```python
from build123d import *

# Parameters (mm, degrees)
SALIENTE_EXTRUIR1_DEPTH = 6
SALIENTE_EXTRUIR4_DEPTH = 141
SALIENTE_EXTRUIR5_DEPTH = 6
REDONDEO10_R            = 2
REDONDEO11_R            = 2
CROQUIS8_R              = 5.2625
CORTAR_EXTRUIR5_DEPTH   = 161
CORTAR_EXTRUIR4_DEPTH   = 45.2325
CROQUIS10_W             = 37.37553938
CROQUIS10_H             = 2.5
SALIENTE_EXTRUIR6_DEPTH = 142
CROQUIS15_W             = 31.064336603
CROQUIS15_H             = 2.5
SALIENTE_EXTRUIR8_DEPTH = 148
CROQUIS16_R             = 1.5
CORTAR_EXTRUIR6_DEPTH   = 156
CORTAR_EXTRUIR7_DEPTH   = 64
CROQUIS19_W             = 16.749018002
CROQUIS19_H             = 43
CORTAR_EXTRUIR9_DEPTH   = 157
REDONDEO12_R            = 10


with BuildPart() as part:
    # Croquis1 → Saliente-Extruir1 (new body)
    with BuildSketch(Plane.XY):
        with BuildLine():
            Line((47.278265355, -15.875), (82.039783357, -15.875))
            Line((82.039783357, -15.875), (82.039783357, 30.125))
            Line((82.039783357, 30.125), (40.807283357, 30.125))
            ThreePointArc((40.807283357, 30.125), (38.163219926, 28.542366774), (38.308878254, 25.464285714))
            ThreePointArc((38.308878254, 25.464285714), (45.409629872, 7.346122436), (44.38367768, -12.086734694))
            ThreePointArc((44.38367768, -12.086734694), (44.89448727, -14.696428571), (47.278265355, -15.875))
        make_face()
    extrude(amount=SALIENTE_EXTRUIR1_DEPTH)

    # Croquis6 → Saliente-Extruir4 (add)
    with BuildSketch(Plane(origin=(0, 0, 0), x_dir=(-1, 0, 0), z_dir=(0, 0, -1))):
        with BuildLine():
            Line((-45.807283357, 27.125), (-40.807283357, 27.125))
            ThreePointArc((-40.807283357, 27.125), (-48.371127473, 7.825217377), (-47.278265355, -12.875))
            Line((-47.278265355, -12.875), (-52.278265355, -12.875))
            Line((-52.278265355, -12.875), (-52.278265355, -15.875))
            Line((-52.278265355, -15.875), (-47.278265355, -15.875))
            ThreePointArc((-47.278265355, -15.875), (-44.89448727, -14.696428571), (-44.38367768, -12.086734694))
            ThreePointArc((-44.38367768, -12.086734694), (-45.409629872, 7.346122436), (-38.308878254, 25.464285714))
            ThreePointArc((-38.308878254, 25.464285714), (-38.163219926, 28.542366774), (-40.807283357, 30.125))
            Line((-40.807283357, 30.125), (-45.807283357, 30.125))
            Line((-45.807283357, 30.125), (-45.807283357, 27.125))
        make_face()
    extrude(amount=SALIENTE_EXTRUIR4_DEPTH)

    # Croquis7 → Saliente-Extruir5 (add)
    with BuildSketch(Plane(origin=(0, 0, -141), x_dir=(-1, 0, 0), z_dir=(0, 0, -1))):
        with BuildLine():
            Line((-82.039783357, 30.125), (-40.807283357, 30.125))
            ThreePointArc((-40.807283357, 30.125), (-38.163219926, 28.542366774), (-38.308878254, 25.464285714))
            ThreePointArc((-38.308878254, 25.464285714), (-45.409629872, 7.346122436), (-44.38367768, -12.086734694))
            ThreePointArc((-44.38367768, -12.086734694), (-44.89448727, -14.696428571), (-47.278265355, -15.875))
            Line((-47.278265355, -15.875), (-82.039783357, -15.875))
            Line((-82.039783357, -15.875), (-82.039783357, 30.125))
        make_face()
    extrude(amount=SALIENTE_EXTRUIR5_DEPTH)

    # Redondeo10
    redondeo10_edges = [part.edges().sort_by_distance(p)[0] for p in [
        (43.307283357, 27.125, 0),
        (48.371127473, 7.825217377, 0),
        (40.807283357, 27.125, -70.5),
        (49.778265355, -12.875, 0),
        (47.278265355, -12.875, -70.5),
        (43.307283357, 27.125, -141),
        (48.371127473, 7.825217377, -141),
        (49.778265355, -12.875, -141),
    ]]
    fillet(redondeo10_edges, radius=REDONDEO10_R)

    # Redondeo11
    redondeo11_edges = [part.edges().sort_by_distance(p)[0] for p in [
        (45.807283357, 28.625, 0),
        (52.278265355, -14.375, 0),
        (52.278265355, -14.375, -141),
        (45.807283357, 28.625, -141),
    ]]
    fillet(redondeo11_edges, radius=REDONDEO11_R)

    # Croquis8 → Cortar-Extruir5 (cut)
    with BuildSketch(Plane(origin=(0, 0, -147), x_dir=(-1, 0, 0), z_dir=(0, 0, -1))):
        with Locations((-57.040765355, -8.1125)):
            Circle(CROQUIS8_R)
        with Locations((-57.040765355, 22.3625)):
            Circle(CROQUIS8_R)
    extrude(amount=-CORTAR_EXTRUIR5_DEPTH, mode=Mode.SUBTRACT)

    # Croquis9 → Cortar-Extruir4 (cut, through all)
    with BuildSketch(Plane(origin=(82.039783357, 0, 0), x_dir=(0, 0, -1), z_dir=(1, 0, 0))):
        with BuildLine():
            Line((138.937038998, 15.125), (138.937038998, -0.914712205))
            Line((138.937038998, -0.914712205), (113.937038998, -0.914712205))
            add(Edge.make_bspline(
                [(113.937038998, 15.125), (103.458760089, 7.301871649), (113.937038998, -0.914712205)],
                knots=[0, 0, 0, 1, 1, 1], degree=2))
            Line((113.937038998, 15.125), (138.937038998, 15.125))
        make_face()
        with BuildLine():
            Line((2.062961002, 15.125), (2.062961002, -0.914712205))
            Line((2.062961002, -0.914712205), (27.062961002, -0.914712205))
            add(Edge.make_bspline(
                [(27.062961002, 15.125), (37.541239911, 7.301871649), (27.062961002, -0.914712205)],
                knots=[0, 0, 0, 1, 1, 1], degree=2))
            Line((27.062961002, 15.125), (2.062961002, 15.125))
        make_face()
    extrude(amount=-CORTAR_EXTRUIR4_DEPTH, mode=Mode.SUBTRACT)

    # Croquis10 → Saliente-Extruir6 (add)
    with BuildSketch(Plane(origin=(0, 0, 0), x_dir=(-1, 0, 0), z_dir=(0, 0, -1))):
        with Locations((-63.352013667, 28.875)):
            Rectangle(CROQUIS10_W, CROQUIS10_H)
    extrude(amount=SALIENTE_EXTRUIR6_DEPTH)

    # Croquis15 → Saliente-Extruir8 (add)
    with BuildSketch(Plane.XY.offset(6)):
        with Locations((66.507615055, -14.625)):
            Rectangle(CROQUIS15_W, CROQUIS15_H)
    extrude(amount=-SALIENTE_EXTRUIR8_DEPTH)

    # Croquis16 → Cortar-Extruir6 (cut)
    with BuildSketch(Plane.XY.offset(6)):
        with Locations((69.039783357, 16.125)):
            Circle(CROQUIS16_R)
        with Locations((68.932075525, -1.717397604)):
            Circle(CROQUIS16_R)
    extrude(amount=-CORTAR_EXTRUIR6_DEPTH, mode=Mode.SUBTRACT)

    # Croquis18 → Cortar-Extruir7 (cut)
    with BuildSketch(Plane(origin=(0, 30.125, 0), x_dir=(1, 0, 0), z_dir=(0, 1, 0))):
        with BuildLine():
            Line((82.039783357, 147), (82.039783357, -6))
            ThreePointArc((82.039783357, -6), (62.701060719, 70.5), (82.039783357, 147))
        make_face()
    extrude(amount=-CORTAR_EXTRUIR7_DEPTH, mode=Mode.SUBTRACT)

    # Croquis19 → Cortar-Extruir9 (cut)
    with BuildSketch(Plane.XY.offset(6)):
        with Locations((73.665274356, 8.625)):
            Rectangle(CROQUIS19_W, CROQUIS19_H)
    extrude(amount=-CORTAR_EXTRUIR9_DEPTH, mode=Mode.SUBTRACT)

    # Redondeo12
    redondeo12_edges = [part.edges().sort_by_distance(p)[0] for p in [
        (65.290765355, -12.875, -144),
        (65.290765355, -12.875, 3),
    ]]
    fillet(redondeo12_edges, radius=REDONDEO12_R)


solid = part.part
```
Verification items for the finished model (mm, model axes). A direction names the side the tool comes from. Give positions to 0.01 mm unless a question says otherwise; leave off trailing zeros. Order: outer loops, then holes, each group sorted by start corner. A loop starts at its lowest first (then second) coordinate and runs counter-clockwise, first axis right, second up. Notation, with made-up numbers: (14, 26) -> (22, 26) arc R23 ccw to (22, 61) -> close; hole circle Ø3 at (-11.75, 48). An arc over 180 degrees is marked (long way). One line per item, written item: value.
(1) Sectioned sample at C-C on x = 60. Record the cut outline in (y, z) (3 decimals).
Final values:
outline: (-15.875, -147) -> (-12.464, -147) -> (-12.464, -141) -> (-13.375, -141) -> (-13.375, 0) -> (-12.464, 0) -> (-12.464, 6) -> (-15.875, 6) -> close; (-3.761, -147) -> (18.011, -147) -> (18.011, -141) -> (-3.761, -141) -> close; (-3.761, 0) -> (18.011, 0) -> (18.011, 6) -> (-3.761, 6) -> close; (26.714, -147) -> (30.125, -147) -> (30.125, 6) -> (26.714, 6) -> (26.714, 0) -> (27.625, 0) -> (27.625, -141) -> (26.714, -141) -> close
(2) Gauge pin test, flat ends, axial feed: pin 1 (17 mm diameter, centred on x = 57.04, y = 22.36, fed in from +Z); pin 2 (1 mm diameter, centred on y = 7.5, z = -78.5, fed in from +X); pin 3 (3.5 mm diameter, centred on x = 45, z = -127, fed in from -Y); pin 4 (3 mm diameter, centred on x = 79.5, z = -143.5, fed in from +Y) (3 decimals). Record the tip position at first contact, or that the pin passes through.
Final values:
pin 1: z = 6
pin 2: x = 48.5
pin 3: y = -15.83
pin 4: y = -12.875
(3) Sectioned sample at D-D on z = -56.5. Record the cut outline in (x, y) (3 decimals), then the cut area to 3 significant figures.
Final values:
outline: (38.309, 25.464) arc R46 cw to (44.384, -12.087) arc R3 ccw to (47.278, -15.875) -> (63.311, -15.875) -> (63.311, -13.375) -> (52.278, -13.375) -> (52.278, -12.875) -> (49.827, -12.875) arc R2 cw to (47.873, -10.449) arc R49 ccw to (42.641, 24.14) arc R2 cw to (44.382, 27.125) -> (45.807, 27.125) -> (45.807, 27.625) -> (63.311, 27.625) -> (63.311, 30.125) -> (40.807, 30.125) arc R3 ccw to start
area: 245 mm^2
(4) Sectioned sample at B-B on z = -21.5. Record the cut outline in (x, y) (3 decimals), then the cut area to 3 significant figures.
Final values:
outline: (38.309, 25.464) arc R46 cw to (43.442, 15.125) -> (46.607, 15.125) arc R49 ccw to (42.641, 24.14) arc R2 cw to (44.382, 27.125) -> (45.807, 27.125) -> (45.807, 27.625) -> (65.291, 27.625) -> (65.291, 30.125) -> (40.807, 30.125) arc R3 ccw to start; (44.384, -12.087) arc R3 ccw to (47.278, -15.875) -> (70.34, -15.875) -> (70.34, -13.375) -> (52.278, -13.375) -> (52.278, -12.875) -> (49.827, -12.875) arc R2 cw to (47.873, -10.449) arc R49 ccw to (48.991, -0.915) -> (45.991, -0.915) arc R46 cw to start
area: 219 mm^2
(5) Sectioned sample at A-A on x = 73. Record the cut outline in (y, z) (3 decimals).
Final values:
outline: (-15.875, -147) -> (-12.609, -147) -> (-12.609, -141) -> (-13.375, -141) -> (-13.375, -127.155) -> (-15.875, -127.155) -> close; (-15.875, -13.845) -> (-13.375, -13.845) -> (-13.375, 0) -> (-12.609, 0) -> (-12.609, 6) -> (-15.875, 6) -> close
(6) Draft check along Y on faces 1 (the face through (48.41, 7.58, -69.54)), 2 (the face through (57, -15.875, -69)), 3 (the face through (55, 7, -147)). Enter one of: pulls with the +Y half, pulls with the -Y half, needs draft (parallel to the pull), parting line crosses it, or undercut.
Final values:
face 1: undercut
face 2: pulls with the -Y half
face 3: needs draft
(7) Scan lines: line 1 along Y through (x, z) = (52.5, -38) (3 decimals); line 2 along Z through (x, y) = (61.5, 3); line 3 along Y through (x, z) = (51, -95.5) (3 decimals). Record each from-to range of solid material in increasing order. Write a range as [from, to].
Final values:
line 1: [-15.875, -13.375], [27.625, 30.125]
line 2: [-147, -141], [0, 6]
line 3: [-15.875, -12.875], [27.625, 30.125]
(8) Tool access check on faces 4 (the face through (52.2, 20.3, 3)), 5 (the face through (58, 7, -141)), 6 (the face through (65.291, 20, -142)), 7 (the face through (47, 7, -2.063)). Record the directions out of +Z, -Z, +X, -X, +Y, -Y that give a thin tool (end or side, any length) a straight path to the whole face; none if there is none.
Final values:
face 4: +Z, -Z
face 5: +X
face 6: +Z, -Z, +X, +Y
face 7: +X, -X
